```python
from build123d import *

# Parameters (mm, degrees)
SKETCH_1_R          = 8.5
EXTRUDE_1_DEPTH     = 5
SKETCH_2_R          = 9.5
EXTRUDE_2_DEPTH     = 1.2
CUT_EXTRUDE_1_REACH = 8.2
SKETCH_3_R          = 3.5


with BuildPart() as part:
    # 草圖1 → 填料-伸長1 (new body)
    with BuildSketch(Plane.XY):
        Circle(SKETCH_1_R)
    extrude(amount=EXTRUDE_1_DEPTH)

    # 草圖2 → 填料-伸長2 (add)
    with BuildSketch(Plane.XY.offset(5)):
        Circle(SKETCH_2_R)
    extrude(amount=EXTRUDE_2_DEPTH)

    # 草圖3 → 除料-伸長1 (cut, up to next)
    with BuildSketch(Plane.XY.offset(6.2), mode=Mode.PRIVATE) as cut_extrude_1_sk1:
        Circle(SKETCH_3_R)
    cut_extrude_1_tool1 = extrude(cut_extrude_1_sk1.sketch, amount=-CUT_EXTRUDE_1_REACH, mode=Mode.PRIVATE) & part.part
    add(cut_extrude_1_tool1.solids().sort_by_distance((0, 0, 6.2))[0], mode=Mode.SUBTRACT)


solid = part.part
```
Check sheet for the modelled part. Datum: model origin and axes. Units: mm. A direction names the side the tool comes from. Give positions to 0.01 mm unless a question says otherwise; leave off trailing zeros. Write each loop counter-clockwise with the first axis right and the second up, starting at its lowest first coordinate (ties: lowest second). Pieces come first, ordered by that corner, then holes. Notation, with made-up numbers: (-1.5, 80) - (27.5, 80) arc R35 cw to (27.5, 116) - close; hole circle Ø4 at (29, 83). An arc over 180 degrees is marked (long way). Answer as a JSON object with one key per item and string values. Group by question number.
1) Depth check by flat-ended pin: P1, Ø4, axis at x = -0.5, y = -0.5, coming from the +Z side. Enter the tip coordinate at first touch or a pass-through.
2) Sectioned sample at C-C (z = 1.75). Record the cut outline in (x, y), then the cut area to 3 significant figures.
3) Sectioned sample at D-D (y = -5.25). Record the cut outline in (x, z).
4) Thickness scan on probe 1 along Y at (x, z) = (0, 3.5); probe 2 along Z at (x, y) = (7.5, 5.5); probe 3 along X at (y, z) = (2.75, 3.5). Record the ranges inside material, lowest first. Write a range as from..to.
5) Release check for a two-part mould opening along X. For faces 1 (the face through (3.233, -1.341, 3.143)), 2 (the face through (4.57, 7.167, 2.465)), 3 (the face through (4, 0, 0)) record: pulls with the +X half, pulls with the -X half, needs draft (parallel to the pull), parting line crosses it, or undercut.
6) Sectioned sample at A-A (y = 0). Record the cut outline in (x, z).
7) Access from +Z, -Z, +X, -X, +Y, -Y to the whole of each face (thin tool, end or side, straight path). Record for faces 4 (the face through (4, 0, 6.2)), 5 (the face through (-2.2, -8.4, 5)).
Geometry results:
{
 "1": {"P1": "passes through"},
 "2": {"outline": "circle Ø17 at (0, 0); hole circle Ø7 at (0, 0)", "area": "188 mm^2"},
 "3": {"outline": "(-7.92, 5) - (-6.68, 5) - (-6.68, 0) - (6.68, 0) - (6.68, 5) - (7.92, 5) - (7.92, 6.2) - (-7.92, 6.2) - close"},
 "4": {"probe 1": "y = -8.5..-3.5, 3.5..8.5", "probe 2": "z = 5..6.2", "probe 3": "x = -8.04..-2.17, 2.17..8.04"},
 "5": {"face 1": "undercut", "face 2": "parting line crosses it", "face 3": "needs draft"},
 "6": {"outline": "(-9.5, 5) - (-8.5, 5) - (-8.5, 0) - (-3.5, 0) - (-3.5, 6.2) - (-9.5, 6.2) - close; (3.5, 0) - (8.5, 0) - (8.5, 5) - (9.5, 5) - (9.5, 6.2) - (3.5, 6.2) - close"},
 "7": {"face 4": "+Z, +X, -X, +Y, -Y", "face 5": "-Z"}
}
